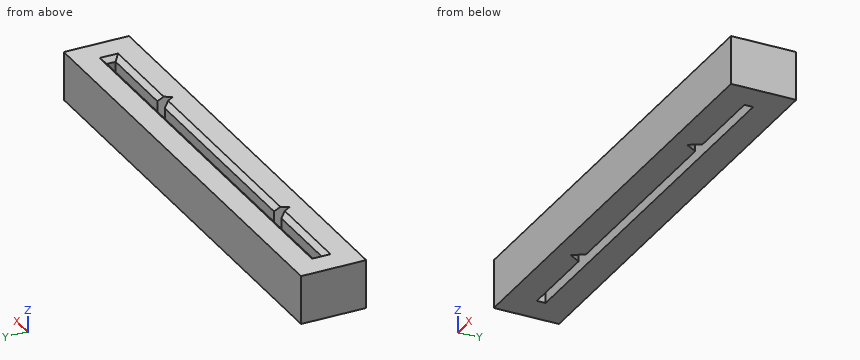
from build123d import *

# Parameters (mm, degrees)
SKETCH_1_W          = 47.8
SKETCH_1_H          = 6.7
EXTRUDE_1_DEPTH     = 5
CUT_EXTRUDE_1_DEPTH = 7.5
CHAMFER_1_SIZE      = 0.5


with BuildPart() as part:
    # Эскиз1 → Бобышка-Вытянуть1 (new body)
    with BuildSketch(Plane(origin=(0, 66.754264805, 0), x_dir=(-1, 0, 0), z_dir=(0, 0, 1))):
        with Locations((0, 66.754264805)):
            Rectangle(SKETCH_1_W, SKETCH_1_H)
    extrude(amount=EXTRUDE_1_DEPTH)

    # Эскиз6 → Вырез-Вытянуть1 (cut)
    with BuildSketch(Plane(origin=(0, 66.754264805, 5), x_dir=(-1, 0, 0), z_dir=(0, 0, 1))):
        Polygon((-20.9, 67.204264805), (-12.5, 67.204264805), (-11.75, 68.404264805), (-11, 67.204264805), (11, 67.204264805), (11.75, 68.404264805), (12.5, 67.204264805), (20.9, 67.204264805), (20.9, 66.304264805), (-20.9, 66.304264805), align=None)
    extrude(amount=-CUT_EXTRUDE_1_DEPTH, mode=Mode.SUBTRACT)

    # Фаска1
    chamfer_1_edges = [part.edges().sort_by_distance(p)[0] for p in [
        (16.7, -0.45, 5),
        (20.9, 0, 5),
        (0, 0.45, 5),
        (-20.9, 0, 5),
        (-16.7, -0.45, 5),
        (0, -0.45, 5),
    ]]
    chamfer(chamfer_1_edges, length=CHAMFER_1_SIZE)


solid = part.part
Geometry: final body of the model. Coordinates: model frame, mm. Give positions to 0.01 mm unless a question says otherwise; leave off trailing zeros. Loops run counter-clockwise (first coordinate to the right, second up) from the corner with the lowest first, then second, coordinate; pieces in that order, holes last. Notation, with made-up numbers: M 62.5,-39 L 73.5,-39 A34 ccw 73.5,0 Z; hole C -23,-14.5 d8. An arc over 180 degrees is marked long. Put each result on its own line as item: value.
1) Material intervals for L1, parallel to Y at x = 18.5, z = 1.1; L2, parallel to X at y = 0, z = 0.65; L3, parallel to X at y = -1, z = 2.35, sorted ascending. Write a range as from..to.
Computed values:
L1: y = -3.35..-0.45, 0.45..3.35
L2: x = -23.9..-20.9, 20.9..23.9
L3: x = -23.9..-12.16, -11.34..11.34, 12.16..23.9
2) Cut plane A-A, the plane y = 0. Return the cut outline in (x, z).
Computed values:
outline: M -23.9,0 L -20.9,0 L -20.9,4.5 L -21.4,5 L -23.9,5 Z; M 20.9,0 L 23.9,0 L 23.9,5 L 21.4,5 L 20.9,4.5 Z
3) Cut plane B-B, the plane x = -10. Return the cut outline in (y, z), plus the area to 4 significant figures.
Computed values:
outline: M -3.35,0 L -0.45,0 L -0.45,4.5 L -0.95,5 L -3.35,5 Z; M 0.45,0 L 3.35,0 L 3.35,5 L 0.95,5 L 0.45,4.5 Z
area: 28.75 mm^2
4) Cut plane C-C, the plane z = 0.7. Return the cut outline in (x, y), plus the area to 3 significant figures.
Computed values:
outline: M -23.9,-3.35 L 23.9,-3.35 L 23.9,3.35 L -23.9,3.35 Z; hole M -20.9,-0.45 L -12.5,-0.45 L -11.75,-1.65 L -11,-0.45 L 11,-0.45 L 11.75,-1.65 L 12.5,-0.45 L 20.9,-0.45 L 20.9,0.45 L -20.9,0.45 Z
area: 281 mm^2
